Here's the drawing with two shaded views (mm, measured from the low corner). I have some questions. A direction names the side the tool comes from. Coordinates: 2 decimals unless noted, no trailing zeros. Order: outer loops, then holes, each group sorted by start corner. A loop starts at its lowest first (then second) coordinate and runs counter-clockwise, first axis right, second up. Notation, with made-up numbers: (-8.75, 0) - (19.25, 0) arc R31 cw to (19.25, 31) - close; hole circle Ø11 at (-5, -3.5). An arc over 180 degrees is marked (long way). Answer as a JSON object with one key per item and string values. Group by question number.
(1) Imagine slicing it at B-B, the plane y = 39. Write out the boundary of the cut face in (x, z), and give its area (3 significant figures).
(2) Imagine slicing it at A-A, the plane x = 6. Write out the boundary of the cut face in (y, z).
(3) Which directions (+Z, -Z, +X, -X, +Y, -Y) give clear straight access to the entire face, cutting with the end or side of a thin tool? Please do the marked faces 1 and 2.
(4) Please list where these lines run through material, in increasing order: probe 1 along X at (y, z) = (61, 16.5); probe 2 along Y at (x, z) = (59, 13.5); probe 3 along Z at (x, y) = (60.5, 82).
(5) Imagine slicing it at C-C, the plane z = 34. Write out the boundary of the cut face in (x, y).
(6) Will these pins go through, and if not, where does the flat tip stop? P1, Ø9.5, axis at x = 55.5, y = 40.5, coming from the +Z side; P2, Ø10, axis at x = 52, z = 20.5, coming from the +Y side.
(7) We'd pull the mould along X, two halves only. Please class the marked faces 3, 4 and 5: pulls with the +X half, pulls with the -X half, needs draft (parallel to the pull), parting line crosses it, or undercut.
(8) Imagine slicing it at D-D, the plane x = 37.5. Write out the boundary of the cut face in (y, z), and give its area (3 significant figures).
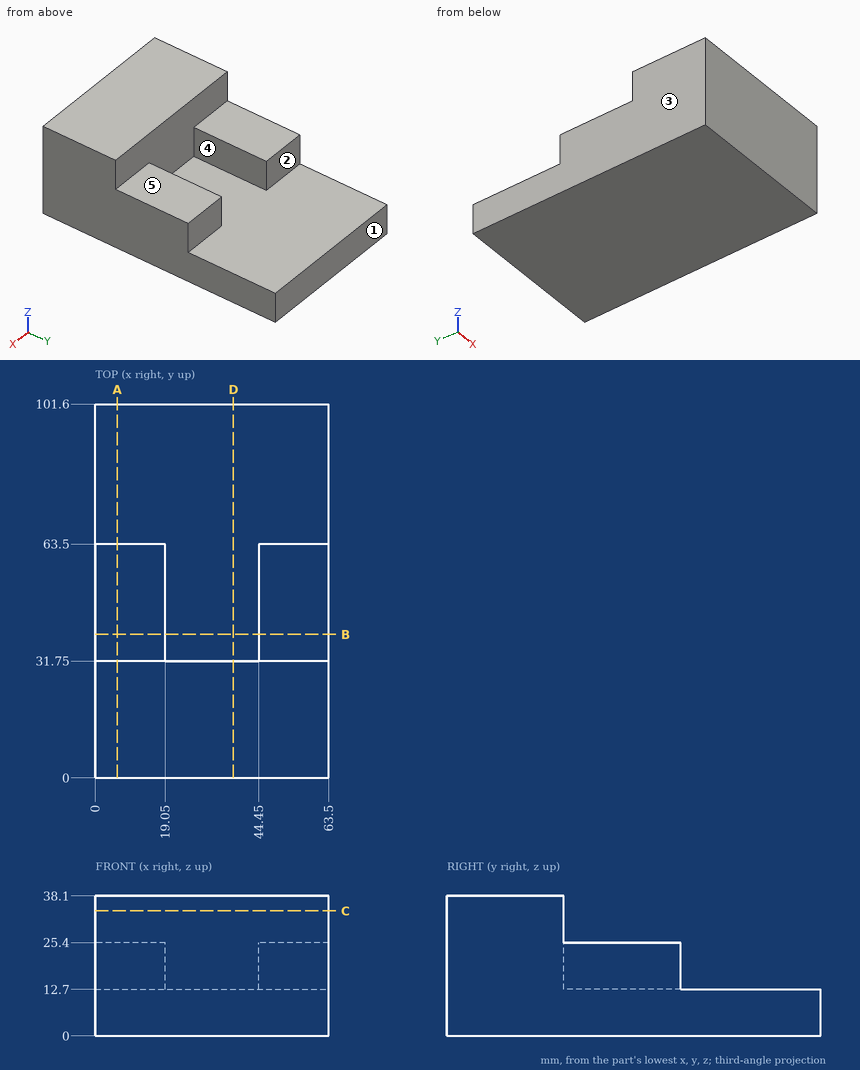
Result set:
{
 "1": {"outline": "(0, 0) - (63.5, 0) - (63.5, 25.4) - (44.45, 25.4) - (44.45, 12.7) - (19.05, 12.7) - (19.05, 25.4) - (0, 25.4) - close", "area": "1,290 mm^2"},
 "2": {"outline": "(0, 0) - (101.6, 0) - (101.6, 12.7) - (63.5, 12.7) - (63.5, 25.4) - (31.75, 25.4) - (31.75, 38.1) - (0, 38.1) - close"},
 "3": {"face 1": "+Z, -Z, +X, -X, +Y", "face 2": "+Z, +X, -X, +Y"},
 "4": {"probe 1": "x = 0 to 19.05, 44.45 to 63.5", "probe 2": "y = 0 to 63.5", "probe 3": "z = 0 to 12.7"},
 "5": {"outline": "(0, 0) - (63.5, 0) - (63.5, 31.75) - (0, 31.75) - close"},
 "6": {"P1": "stops at z = 25.4", "P2": "stops at y = 63.5"},
 "7": {"face 3": "pulls with the -X half", "face 4": "undercut", "face 5": "needs draft"},
 "8": {"outline": "(0, 0) - (101.6, 0) - (101.6, 12.7) - (31.75, 12.7) - (31.75, 38.1) - (0, 38.1) - close", "area": "2,100 mm^2"}
}
